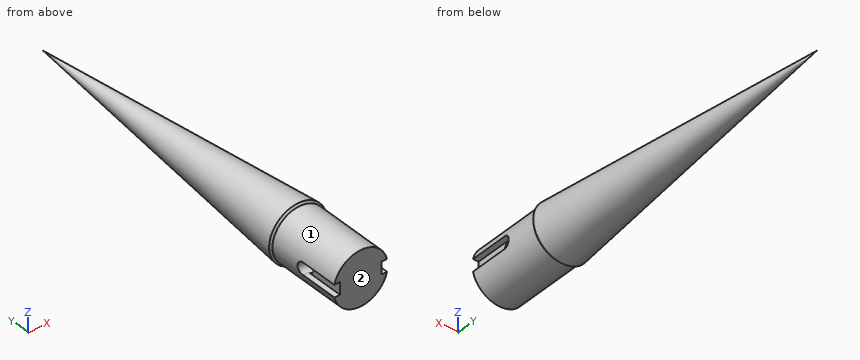
```python
from build123d import *

# Parameters (mm, degrees)
SKETCH1_R               = 8.895
BOSS_EXTRUDE1_DEPTH     = 25
CUT_EXTRUDE1_DEPTH      = 12.5
SKETCH3_R               = 1.984375
CUT_EXTRUDE2_DEPTH      = 9.895
CUT_EXTRUDE2_DEPTH_BACK = 9.895
CHAMFER1_SIZE           = 0.6


with BuildPart() as part:
    # Sketch1 → Boss-Extrude1 (new body)
    with BuildSketch(Plane(origin=(0, 0, 0), x_dir=(1, 0, 0), z_dir=(0, 1, 0))):
        Circle(SKETCH1_R)
    extrude(amount=-BOSS_EXTRUDE1_DEPTH)

    # Sketch2 → Cut-Extrude1 (cut)
    with BuildSketch(Plane.XZ.offset(25)):
        with BuildLine():
            Line((-6.83125, 1.984375), (-6.83125, -1.984375))
            Line((-6.83125, -1.984375), (-8.670829306, -1.984375))
            ThreePointArc((-8.670829306, -1.984375), (-8.895, 0), (-8.670829306, 1.984375))
            Line((-8.670829306, 1.984375), (-6.83125, 1.984375))
        make_face()
    cut_extrude1 = extrude(amount=-CUT_EXTRUDE1_DEPTH, mode=Mode.SUBTRACT)

    # Mirror1: Cut-Extrude1 across plane
    add(cut_extrude1.mirror(Plane(origin=(0, 0, 0), x_dir=(0, 0, 1), z_dir=(1, 0, 0))), mode=Mode.SUBTRACT)

    # Sketch3 → Cut-Extrude2 (cut, two sides)
    with BuildSketch(Plane(origin=(0, 0, 0), x_dir=(0, 0, -1), z_dir=(1, 0, 0))) as cut_extrude2_sk:
        with Locations((0, -12.5)):
            Circle(SKETCH3_R)
    extrude(amount=CUT_EXTRUDE2_DEPTH, mode=Mode.SUBTRACT)
    extrude(cut_extrude2_sk.sketch, amount=-CUT_EXTRUDE2_DEPTH_BACK, mode=Mode.SUBTRACT)

    # Sketch4 → Revolve1 (revolve)
    with BuildSketch(Plane.XY):
        Polygon((0, 0), (9.5, 0), (0, 101.6), align=None)
    revolve(axis=Axis((0, 101.6, 0), (0, -1, 0)))

    # Chamfer1
    chamfer1_edges = [part.edges().sort_by_distance(p)[0] for p in [
        (-8.895, 0, 0),
    ]]
    chamfer(chamfer1_edges, length=CHAMFER1_SIZE)


solid = part.part
```
Verification items for the finished model (mm, model axes). Face numbers are marked on the shaded views. A direction names the side the tool comes from. Give positions to 0.01 mm unless a question says otherwise; leave off trailing zeros. Loops run counter-clockwise (first coordinate to the right, second up) from the corner with the lowest first, then second, coordinate; pieces in that order, holes last. Notation, with made-up numbers: M 75,-1 L 127,-1 A21 ccw 127,28 Z; hole C 66.25,27.5 d6. An arc over 180 degrees is marked long. Return JSON: item names as keys, results as strings.
1) Tool access check on the marked faces 1 and 2. Record the directions out of +Z, -Z, +X, -X, +Y, -Y that give a thin tool (end or side, any length) a straight path to the whole face; none if there is none.
Findings:
{"face 1": "-Y", "face 2": "+Z, -Z, +X, -X, -Y"}
2) Section check A-A, the plane y = 60.5. Enter the section's corners in (x, z).
Findings:
{"outline": "C 0,0 d7.69"}
3) Gauge pin test, flat ends, axial feed: P1, Ø5, axis at y = -12.5, z = 0, coming from the -X side (3 decimals); P2, Ø2, axis at y = -19.5, z = 0, coming from the +X side; P3, Ø2, axis at x = -7.5, y = -20.5, coming from the +Z side. Record the tip position at first contact, or that the pin passes through.
Findings:
{"P1": "stops at x = -8.895", "P2": "stops at x = 6.83", "P3": "stops at z = 6.07"}
4) Section check B-B, the plane y = 16. Enter the section's corners in (x, z).
Findings:
{"outline": "C 0,0 d16.01"}
5) Material ranges on L1, parallel to Z at x = -4.25, y = -12.5; L2, parallel to Z at x = -2, y = -10; L3, parallel to Z at x = 4, y = -12.5, recorded low to high. Write a range as [from, to].
Findings:
{"L1": "z = [-7.81, -1.98], [1.98, 7.81]", "L2": "z = [-8.67, 8.67]", "L3": "z = [-7.94, -1.98], [1.98, 7.94]"}
